from build123d import *

# Parameters (mm, degrees)
F0_R     = 5
F1_DEPTH = 5
F2_SIZE  = 3
F3_R     = 2
F4_DEPTH = 45
F5_SIZE  = 2
F7_DEPTH = 1


with BuildPart() as f1:
    # F0 (on Front) → F1 (new body)
    with BuildSketch(Plane.XZ):
        Circle(F0_R)
    extrude(amount=F1_DEPTH)

    # F2
    f2_edges = [f1.edges().sort_by_distance(p)[0] for p in [
        (-5, 0, 0),
    ]]
    chamfer(f2_edges, length=F2_SIZE)

    # F3 (on face) → F4 (join)
    with BuildSketch(Plane(origin=(0, 0, 0), x_dir=(-1, 0, 0), z_dir=(0, 1, 0))):
        Circle(F3_R)
    extrude(amount=F4_DEPTH)

    # F5
    f5_edges = [f1.edges().sort_by_distance(p)[0] for p in [
        (2, 45, 0),
    ]]
    chamfer(f5_edges, length=F5_SIZE)

    # F6 (on face) → F7 (cut)
    with BuildSketch(Plane.XZ.offset(5)):
        Polygon((1, 3), (-1, 3), (-1, 1), (-3, 1), (-3, -1), (-1, -1), (-1, -3), (1, -3), (1, -1), (3, -1), (3, 1), (1, 1), align=None)
    extrude(amount=-F7_DEPTH, mode=Mode.SUBTRACT)


solid = f1.part
The model under review builds one solid part; all positions refer to its coordinate system, in mm. A direction names the side the tool comes from. Round coordinates to 2 decimals unless told otherwise and drop trailing zeros. Loops run counter-clockwise (first coordinate to the right, second up) from the corner with the lowest first, then second, coordinate; pieces in that order, holes last. Notation, with made-up numbers: (68.25, 0) -> (121.25, 0) arc R14 ccw to (121.25, 9) -> close; hole circle Ø8 at (31.25, -10). An arc over 180 degrees is marked (long way). One line per question, with ' | ' between items. Start each with the question number.
Item 1: For pin 1 (6 mm diameter, centred on y = 38.5, z = -3.5, fed in from -X); pin 2 (0.8 mm diameter, centred on y = -4.5, z = 2, fed in from +X); pin 3 (0.8 mm diameter, centred on x = 2, y = -4.5, fed in from +Z), all flat-tipped, find the tip position at first contact; note any pin that passes through.
Item 2: Add section A-A, the plane y = 9.5. Write out the cut boundary in (x, z).
Item 3: Wall thickness on line 1 along Z through (x, y) = (0, 29); line 2 along Y through (x, z) = (-3.5, 0.25); line 3 along X through (y, z) = (29.5, -0.25): over which ranges is each line inside the solid? List them lowest first. Write a range as [from, to].
Item 4: Draft analysis for pull direction Z (two halves, no side actions). For faces 1 (the face through (-1.2, -5, 1.2)), 2 (the face through (0, 21, -2)), 3 (the face through (-1, -4.5, -2)), state which applies: +Z half, -Z half, draft (parallel to the pull), parting line (faces both ways), or undercut.
Item 5: Machinability: for faces 4 (the face through (-0.465, -0.146, -2.095)), 5 (the face through (3, -4.5, 0)), which of the approach directions +Z, -Z, +X, -X, +Y, -Y give a long, thin tool a straight path to every point of the face, cutting with its end or side? Answer none if there is none.
Return value:
1) pin 1: stops at x = -1.94 | pin 2: stops at x = 4.74 | pin 3: stops at z = 4.74
2) outline: circle Ø4 at (0, 0)
3) line 1: z = [-2, 2] | line 2: y = [-5, -1.51] | line 3: x = [-1.98, 1.98]
4) face 1: draft | face 2: parting line | face 3: undercut
5) face 4: +Y | face 5: -Y
